For this review, take the finished solid that the model builds, in its own axes (mm). A direction names the side the tool comes from. Coordinates: 2 decimals unless noted, no trailing zeros. Write each loop counter-clockwise with the first axis right and the second up, starting at its lowest first coordinate (ties: lowest second). Pieces come first, ordered by that corner, then holes. Notation, with made-up numbers: (84, 77.5) -> (110, 77.5) arc R19 ccw to (110, 113.5) -> close; hole circle Ø4 at (21, 4.5). An arc over 180 degrees is marked (long way). One line per item, written item: value. Start each with the question number.
1) Mouldability with a two-part tool opening along Y and no side actions: class faces 1 (the flat face through (18.63, -11.99, 1.97)), 2 (the cylindrical face through (294.3, -4.4, 2)), 3 (the cylindrical face through (9.252, 2.914, 1.972)), 4 (the flat face through (-1.31, 21.99, 1.97)) as released by +Y, released by -Y, zero draft, split by the parting line, or undercut.
2) Machinability: for faces 5 (the flat face through (157, 7, 0)), 6 (the flat face through (164.311, -18.136, 1.972)), which of the approach directions +Z, -Z, +X, -X, +Y, -Y give a long, thin tool a straight path to every point of the face, cutting with its end or side? Answer none if there is none.
3) Add section D-D (x = 226.5). State the section outline as (y, z) points.
4) For probe 1 along Y at (x, z) = (300, 1.1); probe 2 along Y at (x, z) = (319, 2.45); probe 3 along X at (y, z) = (13.5, 0.2), list the stretches that pass through material, from the lowest coordinate up. Write a range as from..to.
5) Add section B-B (z = 1.1). State how many separate pieces and enclosed holes the cut face has, and give its area (3 significant figures).
6) For pin 1 Ø1.5 at (y, z) = (1, 1) entering from -X; pin 2 Ø2 at (x, z) = (60.5, 1.5) entering from +Y, all flat-tipped, find the tip position at first contact; note any pin that passes through.
7) Add section C-C (x = 152.5). State the section outline as (y, z) points, and give its area (3 significant figures).
8) Add section A-A (x = 0). State the section outline as (y, z) points.
from build123d import *

# Parameters (mm, degrees)
SKETCH_1_R      = 9.7
SKETCH_1_R_2    = 7.2
SKETCH_1_R_3    = 2
EXTRUDE_1_DEPTH = 4


with BuildPart() as part:
    # 草图1 → 凸台-拉伸1 (new body)
    with BuildSketch(Plane.XY):
        with BuildLine():
            Line((-9.85, 17.060700455), (7.470508076, 27.060700455))
            Line((7.470508076, 27.060700455), (289.624667154, 27.060700455))
            ThreePointArc((289.624667154, 27.060700455), (328.694852344, 4.11311011), (297.66555963, -28.905888469))
            Line((297.66555963, -28.905888469), (27.170508076, -7.060700455))
            Line((27.170508076, -7.060700455), (9.85, -17.060700455))
            ThreePointArc((9.85, -17.060700455), (-17.060700455, -9.85), (-9.85, 17.060700455))
        make_face()
        Circle(SKETCH_1_R, mode=Mode.SUBTRACT)
        with Locations((300, 0)):
            Circle(SKETCH_1_R_2, mode=Mode.SUBTRACT)
        with Locations((319, 0)):
            Circle(SKETCH_1_R_3, mode=Mode.SUBTRACT)
        with Locations((313.435028843, -13.435028843)):
            Circle(SKETCH_1_R_3, mode=Mode.SUBTRACT)
        with Locations((300, -19)):
            Circle(SKETCH_1_R_3, mode=Mode.SUBTRACT)
        with Locations((286.564971157, -13.435028843)):
            Circle(SKETCH_1_R_3, mode=Mode.SUBTRACT)
        with Locations((281, 0)):
            Circle(SKETCH_1_R_3, mode=Mode.SUBTRACT)
        with Locations((286.564971157, 13.435028843)):
            Circle(SKETCH_1_R_3, mode=Mode.SUBTRACT)
        with Locations((300, 19)):
            Circle(SKETCH_1_R_3, mode=Mode.SUBTRACT)
        with Locations((313.435028843, 13.435028843)):
            Circle(SKETCH_1_R_3, mode=Mode.SUBTRACT)
    extrude(amount=EXTRUDE_1_DEPTH)


solid = part.part
Numbers:
1. face 1: released by -Y
1. face 2: undercut
1. face 3: undercut
1. face 4: released by +Y
2. face 5: -Z, +X, -X, +Y, -Y
2. face 6: +Z, -Z, -Y
3. outline: (-23.16, 0) -> (27.06, 0) -> (27.06, 4) -> (-23.16, 4) -> close
4. probe 1: -29..-21, -17..-7.2, 7.2..17, 21..28.98
4. probe 2: -21.91..-2, 2..21.89
4. probe 3: -14.35..284.57, 288.56..311.44, 315.43..325.65
5. separate pieces: 1
5. enclosed holes: 10
5. area: 14,800 mm²
6. pin 1: x = -19.7
6. pin 2: y = 27.06
7. outline: (-17.18, 0) -> (27.06, 0) -> (27.06, 4) -> (-17.18, 4) -> close
7. area: 177 mm²
8. outline: (-19.7, 0) -> (-9.7, 0) -> (-9.7, 4) -> (-19.7, 4) -> close; (9.7, 0) -> (22.75, 0) -> (22.75, 4) -> (9.7, 4) -> close
